```python
from build123d import *

# Parameters (mm, degrees)
ESQUISSE1_W             = 35
ESQUISSE1_H             = 55
BOSS_EXTRU_1_DEPTH      = 1
ESQUISSE2_W             = 45
ESQUISSE2_H             = 25
BOSS_EXTRU_2_DEPTH      = 2
ESQUISSE3_W             = 5
ESQUISSE3_H             = 10
ENL_V_MAT_EXTRU_1_DEPTH = 2
ESQUISSE5_W             = 25
ESQUISSE5_H             = 20
BOSS_EXTRU_3_DEPTH      = 2
BOSS_EXTRU_4_DEPTH      = 2
SYM_TRIE1_DEPTH         = 4
ESQUISSE7_W             = 13.982195968
ESQUISSE7_H             = 28.94332856
ENL_V_MAT_EXTRU_2_DEPTH = 50
ESQUISSE8_R             = 2.5
ENL_V_MAT_EXTRU_3_DEPTH = 2


# Read off the part's stored shape, not the designer's step: Symétrie1
with BuildPart() as part:
    # Esquisse1 → Boss.-Extru.1 (new body)
    with BuildSketch(Plane(origin=(0, 0, 0), x_dir=(1, 0, 0), z_dir=(0, 1, 0))):
        with Locations((17.5, 27.5)):
            Rectangle(ESQUISSE1_W, ESQUISSE1_H)
    extrude(amount=BOSS_EXTRU_1_DEPTH)

    # Esquisse2 → Boss.-Extru.2 (add)
    with BuildSketch(Plane.ZY):
        with Locations((-27.5, 12.5)):
            Rectangle(ESQUISSE2_W, ESQUISSE2_H)
    extrude(amount=BOSS_EXTRU_2_DEPTH)

    # Esquisse3 → Enlèv. mat.-Extru.1 (cut)
    with BuildSketch(Plane(origin=(0, 0, 0), x_dir=(-1, 0, 0), z_dir=(0, -1, 0))):
        with Locations((-32.5, 50)):
            Rectangle(ESQUISSE3_W, ESQUISSE3_H)
    extrude(amount=-ENL_V_MAT_EXTRU_1_DEPTH, mode=Mode.SUBTRACT)

    # Esquisse5 → Boss.-Extru.3 (add)
    with BuildSketch(Plane(origin=(0, 0, 0), x_dir=(-1, 0, 0), z_dir=(0, -1, 0))):
        with Locations((-22.5, 10)):
            Rectangle(ESQUISSE5_W, ESQUISSE5_H)
    extrude(amount=BOSS_EXTRU_3_DEPTH)

    # Esquisse6 → Boss.-Extru.4 (add)
    with BuildSketch(Plane.XY):
        with BuildLine():
            Line((35, 1), (10, 1))
            Line((10, 1), (10, -15))
            ThreePointArc((10, -15), (22.5, -27.5), (35, -15))
            Line((35, -15), (35, 1))
        make_face()
    extrude(amount=BOSS_EXTRU_4_DEPTH)

    # Symétrie1 outline → Symétrie1 (add)
    with BuildSketch(Plane.XY):
        with BuildLine():
            Line((35, -15), (35, 17))
            ThreePointArc((35, 17), (22.5, 29.5), (10, 17))
            Line((10, 17), (10, -15))
            ThreePointArc((10, -15), (22.5, -27.5), (35, -15))
        make_face()
    extrude(amount=SYM_TRIE1_DEPTH)

    # Esquisse7 → Enlèv. mat.-Extru.2 (cut)
    with BuildSketch(Plane.ZY.offset(-10)):
        with Locations((6.991097984, -16.47166428)):
            Rectangle(ESQUISSE7_W, ESQUISSE7_H)
    extrude(amount=-ENL_V_MAT_EXTRU_2_DEPTH, mode=Mode.SUBTRACT)

    # Esquisse8 → Enlèv. mat.-Extru.3 (cut)
    with BuildSketch(Plane.ZY.offset(2)):
        with Locations((-43.263662177, 12.5)):
            Circle(ESQUISSE8_R)
    extrude(amount=-ENL_V_MAT_EXTRU_3_DEPTH, mode=Mode.SUBTRACT)


solid = part.part
```
Geometry: final body of the model. Coordinates: model frame, mm. A direction names the side the tool comes from. Coordinates: 2 decimals unless noted, no trailing zeros. Order: outer loops, then holes, each group sorted by start corner. A loop starts at its lowest first (then second) coordinate and runs counter-clockwise, first axis right, second up. Notation, with made-up numbers: (61, 88) - (77, 88) arc R24 ccw to (77, 99) - close; hole circle Ø7 at (55.25, -18.5). An arc over 180 degrees is marked (long way). Write each question's results on one line, items separated by ' | '.
(1) Section query B-B, the plane x = 22.5. Return the cut outline in (y, z).
Values found:
outline: (-2, -20) - (0, -20) - (0, -55) - (1, -55) - (1, 0) - (29.5, 0) - (29.5, 4) - (-2, 4) - close
(2) Line query: line 1 (X direction, y = 11, z = -37); line 2 (Y direction, x = 19, z = -30); line 3 (Y direction, x = 31, z = -13). Output: solid intervals per line, ascending. Write a range as [from, to].
Values found:
line 1: x = [-2, 0] | line 2: y = [0, 1] | line 3: y = [-2, 1]
(3) Mould query, pull axis Y, two halves, no side actions, for faces 4 (the face through (23, -2, -8)), 5 (the face through (-1.01, 10.28, -42.11)), 6 (the face through (-2, 13, -28)), 7 (the face through (-1, 25, -28)). Classes: +Y half, -Y half, draft (parallel to the pull), parting line (faces both ways), or undercut.
Values found:
face 4: -Y half | face 5: undercut | face 6: draft | face 7: +Y half
(4) Set-up query: faces 1 (the face through (22, 15, 0)), 2 (the face through (0, 13, -28)), 3 (the face through (23, -1, -20)). Return all of +Z, -Z, +X, -X, +Y, -Y with unobstructed straight access to the full face (end or side cutting, diameter ignored); none if empty.
Values found:
face 1: -Z, +X, -X, +Y | face 2: +Z, -Z, +X, +Y | face 3: -Z, +X, -X, -Y
(5) First-contact query: pin 1 Ø1.6 at (x, y) = (-1.5, 7.5) entering from +Z; pin 2 Ø0.8 at (y, z) = (0.5, -2) entering from -X; pin 3 Ø1 at (x, z) = (22, -6.5) entering from +Y; pin 4 Ø4 at (y, z) = (12.5, -43.26) entering from -X. Flat tips, straight axial feed; report the tip coordinate or a pass-through.
Values found:
pin 1: stops at z = -5 | pin 2: stops at x = 0 | pin 3: stops at y = 1 | pin 4: passes through
(6) Section query C-C, the plane z = -10. Return the cut outline in (x, y), plus the area to 3 significant figures.
Values found:
outline: (-2, 0) - (10, 0) - (10, -2) - (35, -2) - (35, 1) - (0, 1) - (0, 25) - (-2, 25) - close | area: 135 mm²
(7) Section query D-D, the plane y = 21. Return the cut outline in (x, z).
Values found:
outline: (-2, -50) - (0, -50) - (0, -5) - (-2, -5) - close; (10.66, 0) - (34.34, 0) - (34.34, 4) - (10.66, 4) - close
(8) Section query A-A, the plane y = 12.5. Return the cut outline in (x, z).
Values found:
outline: (-2, -50) - (0, -50) - (0, -45.76) - (-2, -45.76) - close; (-2, -40.76) - (0, -40.76) - (0, -5) - (-2, -5) - close; (10, 0) - (35, 0) - (35, 4) - (10, 4) - close
